from build123d import *

# Parameters (mm, degrees)
F3_R     = 6.607149
F4_DEPTH = 44.45


with BuildPart() as f1:
    # F0 (on Front) → F1 (revolve)
    with BuildSketch(Plane.XZ):
        Polygon((-22.225, 12.7), (0, 12.7), (0, 44.196), (-19.05, 44.196), (-19.05, 41.021), (-7.62, 38.1), (-7.62, 22.86), (-22.225, 19.05), align=None)
    revolve(axis=Axis((-1.534584, 0, 0), (1, 0, 0)))

    # F2: F1 across face


with BuildPart() as f1_1:
    add(f1.part)
    add(f1.part.mirror(Plane.YZ))

    # F3 (on Front) → F4 (join)
    with BuildSketch(Plane.XZ):
        Circle(F3_R)
    extrude(amount=F4_DEPTH)


solid = f1_1.part
Input: part model. Units: mm. Frame: model coordinates. A direction names the side the tool comes from. Coordinates: 2 decimals unless noted, no trailing zeros. Loops run counter-clockwise (first coordinate to the right, second up) from the corner with the lowest first, then second, coordinate; pieces in that order, holes last. Notation, with made-up numbers: (39.25, 60) -> (69.25, 60) arc R16 cw to (69.25, 74) -> close; hole circle Ø7 at (50, 15). An arc over 180 degrees is marked (long way). Write each question's results on one line, items separated by ' | '. Start each with the question number.
Q1. Section D-D, the plane x = -10. Return the cut outline in (y, z).
Q2. Section B-B, the plane x = -2. Return the cut outline in (y, z), plus the area to 3 significant figures.
Q3. Pull-direction query (Z, two-part tool) for faces 1 (the cylindrical face through (3.05, -6.27, -5.86)), 2 (the flat face through (-22.225, 4, 12.4)), 3 (the cylindrical face through (3.05, -44.15, -5.86)); classes: released by +Z, released by -Z, zero draft, split by the parting line, or undercut.
Q4. Ray query, line 1 (Z direction, x = -7, y = 0); line 2 (Y direction, x = 8, z = 0); line 3 (Z direction, x = -9, y = 0). Return the intervals inside material, ascending. Write a range as from..to.
Q5. Section C-C, the plane x = 9.5. Return the cut outline in (y, z).
Q6. Pin query (flat end, axial travel): pin 1 (10 mm diameter, centred on y = 9.5, z = -29.5, fed in from -X); pin 2 (6.5 mm diameter, centred on x = -0.5, z = -2.5, fed in from +Y); pin 3 (1.5 mm diameter, centred on x = 8, y = 11, fed in from +Z). Return the tip coordinate at first contact, or that it passes through.
Q7. Reachability of faces 4 (the flat face through (-19.05, 39.1, 12.9)), 5 (the flat face through (0, 0, 0)), 6 (the flat face through (0, -44.45, 0)), 7 (the flat face through (19.05, 39.1, 12.9)) from +Z, -Z, +X, -X, +Y, -Y: full face, straight path, thin tool, end or side. Return the list, or none.
Found:
1) outline: circle Ø88.39 at (0, 0); circle Ø44.48 at (0, 0); hole circle Ø77.42 at (0, 0); hole circle Ø25.4 at (0, 0)
2) outline: (-44.45, -6.3) -> (-43.75, -6.3) arc R44.2 ccw (long way) to (-43.75, 6.3) -> (-44.45, 6.3) -> close; hole (-11.03, -6.3) arc R12.7 ccw (long way) to (-11.03, 6.3) -> (0, 6.3) -> (0, -6.3) -> close | area: 5,790 mm2
3) face 1: undercut | face 2: zero draft | face 3: split by the parting line
4) line 1: -44.2..-12.7, 12.7..44.2 | line 2: -44.2..-38.2, -22.76..-12.7, 12.7..22.76, 38.2..44.2 | line 3: -44.2..-38.45, -22.5..-12.7, 12.7..22.5, 38.45..44.2
5) outline: circle Ø88.39 at (0, 0); circle Ø44.74 at (0, 0); hole circle Ø77.16 at (0, 0); hole circle Ø25.4 at (0, 0)
6) pin 1: x = -7.62 | pin 2: y = 44.2 | pin 3: z = 42.99
7) face 4: -X | face 5: +X, -X | face 6: +Z, -Z, +X, -X, -Y | face 7: +X
